The listing builds one solid part. Answer for the finished solid, in the listing's coordinates (mm). Coordinates: 2 decimals unless noted, no trailing zeros. Loops run counter-clockwise (first coordinate to the right, second up) from the corner with the lowest first, then second, coordinate; pieces in that order, holes last. Notation, with made-up numbers: M 3.25,58 L 49.25,58 A30 cw 49.25,97 Z; hole C 87.5,69.5 d3. An arc over 180 degrees is marked long. Answer as a JSON object with one key per item and string values. Group by question number.
1. A cutting plane is placed at A-A on y = -0.75. Give the vertices of the cut face in (x, z), and give its area (3 significant figures).
2. Determine the mould class of faces 1 (the face through (-2.75, -1, 0)), 2 (the face through (1.394, -1.183, 2.37)), 3 (the face through (-0.27, -1.18, -1.22)) for opening direction Z: released by +Z, released by -Z, zero draft, split by the parting line, or undercut.
3. Given pin 1 (2 mm diameter, centred on x = 0, z = 0, fed in from +Y), flat-ended and moving along its own axis, determine where the tip first touches the part or whether it passes through.
4. Straight lines are drawn through the part: L1, parallel to X at y = -0.3, z = -0.25; L2, parallel to Z at x = 0.5, y = -0.8; L3, parallel to X at y = -1.6, z = 0.5. For each, find the intervals that lie inside material, in ascending order.
from build123d import *

# Parameters (mm, degrees)
F0_R     = 1.25
F1_DEPTH = 2.4


with BuildPart() as f1:
    # F0 (on Front) → F1 (new body)
    with BuildSketch(Plane.XZ):
        Polygon((2.75, -1.587713), (2.75, 1.587713), (0, 3.175426), (-2.75, 1.587713), (-2.75, -1.587713), (0, -3.175426), align=None)
        Circle(F0_R, mode=Mode.SUBTRACT)
    extrude(amount=F1_DEPTH)

    # F2 (on Right) → F3 (revolve, cut)
    with BuildSketch(Plane.YZ):
        with BuildLine():
            add(Edge.make_bspline(
                [(0, -2.675426), (-0.024953, -2.876037), (-0.182256, -3.038666), (-0.3, -3.175426)],
                knots=[0, 0, 0, 0, 0.583095, 0.583095, 0.583095, 0.583095], degree=3))
            Line((-0.3, -3.175426), (0, -3.175426))
            Line((0, -3.175426), (0, -2.675426))
        make_face()
        with BuildLine():
            Line((-2.4, -3.175426), (-2.1, -3.175426))
            add(Edge.make_bspline(
                [(-2.4, -2.675426), (-2.375047, -2.876037), (-2.217744, -3.038666), (-2.1, -3.175426)],
                knots=[0, 0, 0, 0, 0.583095, 0.583095, 0.583095, 0.583095], degree=3))
            Line((-2.4, -2.675426), (-2.4, -3.175426))
        make_face()
    revolve(axis=Axis((0, -1.2, 0), (0, -1, 0)), mode=Mode.SUBTRACT)


solid = f1.part
From the geometry:
{
 "1": {"outline": "M -2.75,-1.59 L 0,-3.18 L 2.75,-1.59 L 2.75,1.59 L 0,3.18 L -2.75,1.59 Z; hole C 0,0 d2.5", "area": "21.3 mm²"},
 "2": {"face 1": "zero draft", "face 2": "released by +Z", "face 3": "undercut"},
 "3": {"pin 1": "passes through"},
 "4": {"L1": "x = -2.75 to -1.22, 1.22 to 2.75", "L2": "z = -2.89 to -1.15, 1.15 to 2.89", "L3": "x = -2.75 to -1.15, 1.15 to 2.75"}
}
